Build history of the part. All positions in model axes, mm. Face numbers are marked on the shaded views. A direction names the side the tool comes from. Coordinates: 2 decimals unless noted, no trailing zeros. Loops run counter-clockwise (first coordinate to the right, second up) from the corner with the lowest first, then second, coordinate; pieces in that order, holes last. Notation, with made-up numbers: (-31, -25) -> (-19, -25) arc R19 ccw to (-19, -21) -> close; hole circle Ø4 at (30, 89). An arc over 180 degrees is marked (long way). One line per item, written item: value. Start each with the question number.
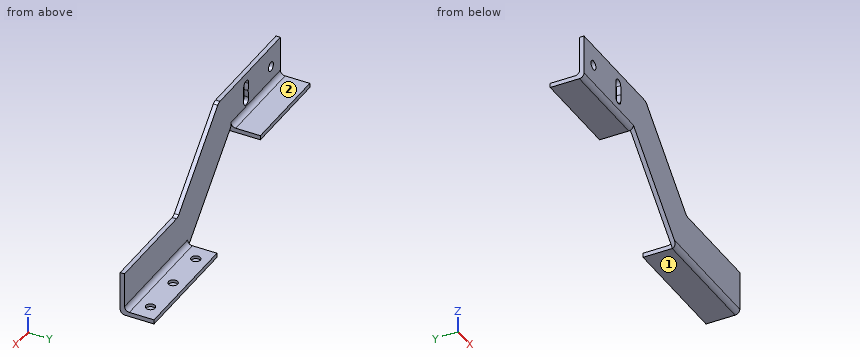
```python
from build123d import *

# Parameters (mm, degrees)
F0_R        = 4.96062
F1_DEPTH    = 4.7625
F2_W        = 31.75
F2_H        = 4.7625
F3_DEPTH    = 127
F4_T1_DEPTH = 127
F4_T3_DEPTH = 152.4
F5_R        = 4.96062
F6_DEPTH    = 3.175
F7_W        = 31.75
F7_H        = 4.7625
F8_DEPTH    = 99.695
F9_R        = 5.08
F11_DEPTH   = 25.4


# Not quite as in the source:
# - a fillet or chamfer that OpenCascade refuses, or shapes differently, is made with other operations: its cross-section is extruded or revolved along the edge and cut away or added


with BuildPart() as f1:
    # F0 (on Front) → F1 (new body)
    with BuildSketch(Plane.XZ):
        with BuildLine():
            Line((-82.55, 82.55), (0, 0))
            Line((0, 0), (127, 0))
            Line((127, 0), (127, 47.625))
            Line((127, 47.625), (22.3571770291, 47.625))
            ThreePointArc((22.3571770291, 47.625), (19.9271372336, 48.1083649686), (17.8670489686, 49.4848719395))
            Line((17.8670489686, 49.4848719395), (-60.9632071525, 128.3151280605))
            ThreePointArc((-60.9632071525, 128.3151280605), (-63.0232954175, 129.6916350314), (-65.4533352131, 130.175))
            Line((-65.4533352131, 130.175), (-187.325, 130.175))
            Line((-187.325, 130.175), (-187.325, 82.55))
            Line((-187.325, 82.55), (-82.55, 82.55))
        make_face()
        with Locations((-168.275, 107.95)):
            Circle(F0_R, mode=Mode.SUBTRACT)
        with BuildLine():
            ThreePointArc((-113.3757178125, 117.6693530802), (-112.7358395418, 112.8283875), (-112.522, 107.95))
            ThreePointArc((-112.522, 107.95), (-112.7358395418, 103.0716125), (-113.3757178125, 98.2306469198))
            ThreePointArc((-113.3757178125, 98.2306469198), (-119.1163255014, 94.2169402337), (-123.1300321875, 99.9575479227))
            ThreePointArc((-123.1300321875, 99.9575479227), (-122.6038452724, 103.9383875), (-122.428, 107.95))
            ThreePointArc((-122.428, 107.95), (-122.6038452724, 111.9616125), (-123.1300321875, 115.9424520773))
            ThreePointArc((-123.1300321875, 115.9424520773), (-119.1163255014, 121.6830597663), (-113.3757178125, 117.6693530802))
        make_face(mode=Mode.SUBTRACT)
    extrude(amount=F1_DEPTH)

    # F2 (on face) → F3 (join)
    with BuildSketch(Plane.YZ.offset(127)):
        with Locations((15.875, 2.38125)):
            Rectangle(F2_W, F2_H)
    extrude(amount=-F3_DEPTH)

    # F4: fillet of radius 5.08 on 2 edges, made by hand

    # F4_s2 → F4_t1 (join)
    with BuildSketch(Plane.YZ):
        with BuildLine():
            ThreePointArc((5.08, 4.7625), (1.4878975516, 6.2503975516), (0, 9.8425))
            Line((0, 9.8425), (0, 4.7625))
            Line((0, 4.7625), (5.08, 4.7625))
        make_face()
    extrude(amount=F4_T1_DEPTH)

    # F4_s4 → F4_t3 (cut)
    with BuildSketch(Plane.YZ.offset(-12.7)):
        with BuildLine():
            ThreePointArc((-4.7625, 5.08), (-3.2746024484, 1.4878975516), (0.3175, 0))
            Line((0.3175, 0), (-4.7625, 0))
            Line((-4.7625, 0), (-4.7625, 5.08))
        make_face()
    extrude(amount=F4_T3_DEPTH, mode=Mode.SUBTRACT)

    # F5 (on face) → F6 (cut)
    with BuildSketch(Plane.XY.offset(4.7625)):
        with Locations((17.79778, 18.42008)):
            Circle(F5_R)
        with Locations((63.51778, 18.42008)):
            Circle(F5_R)
        with Locations((109.23778, 18.42008)):
            Circle(F5_R)
    extrude(amount=-F6_DEPTH, mode=Mode.SUBTRACT)

    # F7 (on face) → F8 (join)
    with BuildSketch(Plane(origin=(-187.325, 0, 0), x_dir=(0, -1, 0), z_dir=(-1, 0, 0))):
        with Locations((-15.875, 84.93125)):
            Rectangle(F7_W, F7_H)
    extrude(amount=-F8_DEPTH)

    # F9
    f9_edges = [f1.edges().sort_by_distance(p)[0] for p in [
        (-134.9375, -4.7625, 82.55),
        (-137.4775, 0, 87.3125),
    ]]
    fillet(f9_edges, radius=F9_R)

    # F10 (on face) → F11 (cut)
    with BuildSketch(Plane.XZ.offset(4.7625)):
        Polygon((-82.5599315833, 82.5599315833), (-87.63, 87.63), (-87.63, 82.5599315833), align=None)
    extrude(amount=-F11_DEPTH, mode=Mode.SUBTRACT)


solid = f1.part
```
Item 1: Band-saw the part on D-D, the plane z = 24. List the corners of the cut face in (x, y), and give its area (3 significant figures).
Item 2: Drop flat-ended pins along their axis: pin 1 Ø6 at (x, y) = (63.52, 18.42) entering from +Z; pin 2 Ø5 at (y, z) = (17.5, 86) entering from +X; pin 3 Ø13.5 at (x, y) = (-113, 23.5) entering from +Z; pin 4 Ø9 at (x, y) = (109.24, 18.42) entering from -Z. Give the stop position or say it passes through.
Item 3: Probe probe 1 along Y at (x, z) = (9, 27); probe 2 along Z at (x, y) = (-90, 26); probe 3 along Z at (x, y) = (33.5, 23). List the from-to ranges inside material, lowest first.
Item 4: Tool access for the marked faces 1 and 2: list every direction of +Z, -Z, +X, -X, +Y, -Y with a clear straight run to the whole face (end or side of a thin tool).
Worked out:
1. outline: (-24, -4.76) -> (127, -4.76) -> (127, 0) -> (-24, 0) -> close
1. area: 719 mm²
2. pin 1: stops at z = 1.59
2. pin 2: stops at x = -87.63
2. pin 3: stops at z = 87.31
2. pin 4: stops at z = 0
3. probe 1: y = -4.76 to 0
3. probe 2: z = 82.55 to 87.31
3. probe 3: z = 0 to 4.76
4. face 1: -Z, +X, -X, +Y, -Y
4. face 2: +Z, +X, -X, +Y
